Source: CAD feature listing. Evaluate the final solid. Frame: model axes, mm. Face numbers are marked on the shaded views. A direction names the side the tool comes from. Round coordinates to 2 decimals unless told otherwise and drop trailing zeros. Write each loop counter-clockwise with the first axis right and the second up, starting at its lowest first coordinate (ties: lowest second). Pieces come first, ordered by that corner, then holes. Notation, with made-up numbers: (22, 43.25) -> (73, 43.25) arc R8 ccw to (73, 55.25) -> close; hole circle Ø8 at (54.5, -8). An arc over 180 degrees is marked (long way). Return JSON: item names as keys, results as strings. Group by question number.
from build123d import *

# Parameters (mm, degrees)
SKETCH1_W                 = 5.5
SKETCH1_H                 = 39.3
BOSS_EXTRUDE1_DEPTH       = 1
SKETCH3_W                 = 15.5
SKETCH3_H                 = 26
BOSS_EXTRUDE5_DEPTH       = 2
SKETCH3_2_W               = 15.5
SKETCH3_2_H               = 26
BOSS_EXTRUDE6_DEPTH       = 2
CUT_EXTRUDE5_DEPTH        = 30.062174729
CUT_EXTRUDE5_DEPTH_BACK   = 14.5
SKETCH10_W                = 2
SKETCH10_H                = 24
SKETCH11_W                = 9.5
SKETCH11_H                = 16
CUT_EXTRUDE7_DEPTH        = 10
F_2_0MM_DOWEL_HOLE1_D     = 2
F_2_0MM_DOWEL_HOLE1_DEPTH = 1
SKETCH15_W                = 3
SKETCH15_H                = 0.5
BOSS_EXTRUDE7_DEPTH       = 0.5


with BuildPart() as part:
    # Sketch1 → Boss-Extrude1 (new body)
    with BuildSketch(Plane.XY):
        Rectangle(SKETCH1_W, SKETCH1_H)
    extrude(amount=BOSS_EXTRUDE1_DEPTH)

    # Sketch3 → Boss-Extrude5 (add, symmetric)
    with BuildSketch(Plane.XY.offset(1)):
        with Locations((0, 11.4)):
            Rectangle(SKETCH3_W, SKETCH3_H)
    extrude(amount=BOSS_EXTRUDE5_DEPTH, both=True)

    # Sketch3<2> → Boss-Extrude6 (add)
    with BuildSketch(Plane.XY.offset(1)):
        with Locations((0, 11.4)):
            Rectangle(SKETCH3_2_W, SKETCH3_2_H)
    extrude(amount=BOSS_EXTRUDE6_DEPTH)

    # Sketch10 → Cut-Extrude5 (cut, two sides: drawn at the far end of the back side and taken through both)
    with BuildSketch(Plane(origin=(7.75, 0, 0), x_dir=(0, 0, -1), z_dir=(1, 0, 0)).offset(-CUT_EXTRUDE5_DEPTH_BACK)):
        with Locations((-1, 11.4)):
            Rectangle(SKETCH10_W, SKETCH10_H)
    extrude(amount=CUT_EXTRUDE5_DEPTH + CUT_EXTRUDE5_DEPTH_BACK, mode=Mode.SUBTRACT)

    # Sketch11 → Cut-Extrude7 (cut)
    with BuildSketch(Plane.XY.offset(3)):
        with Locations((0, 11.4)):
            Rectangle(SKETCH11_W, SKETCH11_H)
    extrude(amount=-CUT_EXTRUDE7_DEPTH, mode=Mode.SUBTRACT)

    # Ø2.0mm Dowel Hole1
    with Locations(Plane(origin=(-0.25, 21.9, 3), x_dir=(1, 0, 0), z_dir=(0, 0, 1))):
        with Locations((0, 0), (0, -21)):
            Hole(F_2_0MM_DOWEL_HOLE1_D / 2, depth=F_2_0MM_DOWEL_HOLE1_DEPTH)

    # Sketch15 → Boss-Extrude7 (add)
    with BuildSketch(Plane.XY.offset(3)):
        with Locations((6.25, 14.4)):
            Rectangle(SKETCH15_W, SKETCH15_H)
        with Locations((6.25, 8.4)):
            Rectangle(SKETCH15_W, SKETCH15_H)
    extrude(amount=BOSS_EXTRUDE7_DEPTH)


solid = part.part
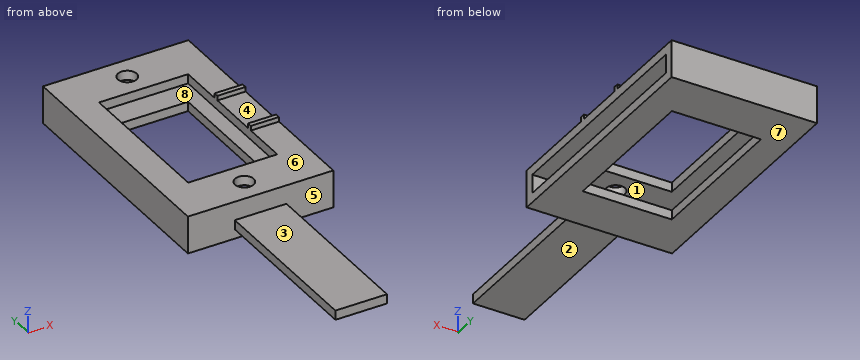
Item 1: Cut plane B-B on x = -0.25. Output: boundary loops of the cut face in (y, z), and give its area (4 significant figures).
Item 2: Cut plane C-C on y = 21.9. Output: boundary loops of the cut face in (x, z).
Item 3: Cut plane A-A on y = 12.5. Output: boundary loops of the cut face in (x, z), and give its area (3 significant figures).
Item 4: Set-up query: the marked faces 1, 2, 3 and 4. Return all of +Z, -Z, +X, -X, +Y, -Y with unobstructed straight access to the full face (end or side cutting, diameter ignored); none if empty.
Item 5: Cut plane D-D on x = -3.5. Output: boundary loops of the cut face in (y, z).
Item 6: First-contact query: pin 1 Ø2.5 at (x, y) = (6, 10) entering from +Z; pin 2 Ø0.8 at (x, z) = (0, 2.5) entering from -Y; pin 3 Ø7 at (x, y) = (-1.5, 6.5) entering from -Z; pin 4 Ø0.5 at (y, z) = (-12.5, 0.5) entering from -X. Flat tips, straight axial feed; report the tip coordinate or a pass-through.
Item 7: Material intervals for probe 1 along Y at (x, z) = (-0.25, 2.3); probe 2 along Y at (x, z) = (4, 1.9); probe 3 along Z at (x, y) = (4.25, 0.5), sorted ascending.
Item 8: Pull-direction query (Z, two-part tool) for the marked faces 5, 6, 7 and 8; classes: +Z half, -Z half, draft (parallel to the pull), parting line (faces both ways), or undercut.
Here are the results:
{
 "1": {"outline": "(-19.65, 0) -> (-1.6, 0) -> (-1.6, -1) -> (3.4, -1) -> (3.4, 0) -> (-0.6, 0) -> (-0.6, 2) -> (-0.1, 2) -> (-0.1, 3) -> (-1.6, 3) -> (-1.6, 1) -> (-19.65, 1) -> close; (1.9, 2) -> (3.4, 2) -> (3.4, 3) -> (1.9, 3) -> close; (19.4, -1) -> (24.4, -1) -> (24.4, 3) -> (22.9, 3) -> (22.9, 2) -> (23.4, 2) -> (23.4, 0) -> (19.4, 0) -> close; (19.4, 2) -> (20.9, 2) -> (20.9, 3) -> (19.4, 3) -> close", "area": "38.05 mm^2"},
 "2": {"outline": "(-7.75, -1) -> (7.75, -1) -> (7.75, 0) -> (-6.75, 0) -> (-6.75, 2) -> (-1.25, 2) -> (-1.25, 3) -> (-7.75, 3) -> close; (0.75, 2) -> (7.75, 2) -> (7.75, 3) -> (0.75, 3) -> close"},
 "3": {"outline": "(-7.75, -1) -> (-4.75, -1) -> (-4.75, 0) -> (-6.75, 0) -> (-6.75, 2) -> (-4.75, 2) -> (-4.75, 3) -> (-7.75, 3) -> close; (4.75, -1) -> (7.75, -1) -> (7.75, 0) -> (4.75, 0) -> close; (4.75, 2) -> (7.75, 2) -> (7.75, 3) -> (4.75, 3) -> close", "area": "14.0 mm^2"},
 "4": {"face 1": "+X", "face 2": "-Z, +X, -X, -Y", "face 3": "+Z, +X, -X, -Y", "face 4": "+Z, +X, -X"},
 "5": {"outline": "(-1.6, -1) -> (3.4, -1) -> (3.4, 0) -> (-0.6, 0) -> (-0.6, 2) -> (3.4, 2) -> (3.4, 3) -> (-1.6, 3) -> close; (19.4, -1) -> (24.4, -1) -> (24.4, 3) -> (19.4, 3) -> (19.4, 2) -> (23.4, 2) -> (23.4, 0) -> (19.4, 0) -> close"},
 "6": {"pin 1": "stops at z = 3", "pin 2": "stops at y = -1.6", "pin 3": "stops at z = -1", "pin 4": "stops at x = -2.75"},
 "7": {"probe 1": "y = -1.6 to -0.1, 1.9 to 3.4, 19.4 to 20.9, 22.9 to 24.4", "probe 2": "y = -1.6 to -0.6, 23.4 to 24.4", "probe 3": "z = -1 to 0, 2 to 3"},
 "8": {"face 5": "draft", "face 6": "+Z half", "face 7": "-Z half", "face 8": "undercut"}
}
